Source: CAD feature listing. Evaluate the final solid. Frame: model axes, mm. A direction names the side the tool comes from. Round coordinates to 2 decimals unless told otherwise and drop trailing zeros. Write each loop counter-clockwise with the first axis right and the second up, starting at its lowest first coordinate (ties: lowest second). Pieces come first, ordered by that corner, then holes. Notation, with made-up numbers: M 25.25,-3.5 L 81.25,-3.5 A9 cw 81.25,2.5 Z; hole C 52,39 d8. An arc over 180 degrees is marked long. Answer in a Markdown table with one row per item.
from build123d import *

# Parameters (mm, degrees)
BOSS_EXTRUDE1_DEPTH = 20


with BuildPart() as part:
    # Sketch1 → Boss-Extrude1 (new body)
    with BuildSketch(Plane(origin=(0, 10, 0), x_dir=(1, 0, 0), z_dir=(0, 1, 0))):
        with BuildLine():
            Line((324.62395369, 187.030739377), (-95.643756342, 187.030739377))
            Line((-95.643756342, 187.030739377), (-95.643756342, -106.347051638))
            Line((-95.643756342, -106.347051638), (-65.143756342, -106.347051638))
            Line((-65.143756342, -106.347051638), (-65.143756342, -33.38491726))
            Line((-65.143756342, -33.38491726), (-65.143756342, 39.577217118))
            Line((-65.143756342, 39.577217118), (-65.143756342, 113.493168526))
            ThreePointArc((-65.143756342, 113.493168526), (-65.012374488, 114.20609645), (-64.635490117, 114.825358582))
            Line((-64.635490117, 114.825358582), (-32.303983997, 151.028901364))
            ThreePointArc((-32.303983997, 151.028901364), (-25.878259507, 159.012700556), (-18.37604631, 152.030739377))
            ThreePointArc((-18.37604631, 152.030739377), (-20.50295437, 147.005505557), (-25.591182009, 145.034046113))
            Line((-25.591182009, 145.034046113), (-55.635490117, 111.391617273))
            ThreePointArc((-55.635490117, 111.391617273), (-56.012374488, 110.772355142), (-56.143756342, 110.059427218))
            Line((-56.143756342, 110.059427218), (-56.143756342, 54.882804578))
            ThreePointArc((-56.143756342, 54.882804578), (-54.925540994, 53.041931753), (-52.754943584, 53.443638458))
            Line((-52.754943584, 53.443638458), (-29.527180359, 75.858711639))
            ThreePointArc((-29.527180359, 75.858711639), (-22.786771169, 83.339716759), (-15.544017337, 76.34392727))
            ThreePointArc((-15.544017337, 76.34392727), (-17.860778034, 71.141305851), (-23.277522947, 69.382464097))
            Line((-23.277522947, 69.382464097), (-55.5325691, 38.255953421))
            ThreePointArc((-55.5325691, 38.255953421), (-55.984629167, 37.598571952), (-56.143756342, 36.816787301))
            Line((-56.143756342, 36.816787301), (-56.143756342, -16.173695516))
            ThreePointArc((-56.143756342, -16.173695516), (-54.850365584, -18.044712186), (-52.643052963, -17.495773188))
            Line((-52.643052963, -17.495773188), (-32.564764827, 5.295289321))
            ThreePointArc((-32.564764827, 5.295289321), (-26.169560776, 13.324151457), (-18.643756342, 6.34392727))
            ThreePointArc((-18.643756342, 6.34392727), (-20.753710482, 1.335189757), (-25.811599623, -0.6540602))
            Line((-25.811599623, -0.6540602), (-55.644459721, -34.517633364))
            ThreePointArc((-55.644459721, -34.517633364), (-56.014773012, -35.133101793), (-56.143756342, -35.839711035))
            Line((-56.143756342, -35.839711035), (-56.143756342, -106.347051638))
            Line((-56.143756342, -106.347051638), (39.856243658, -106.347051638))
            Line((39.856243658, -106.347051638), (39.856243658, -33.38491726))
            Line((39.856243658, -33.38491726), (39.856243658, 39.577217118))
            Line((39.856243658, 39.577217118), (39.856243658, 113.493168526))
            ThreePointArc((39.856243658, 113.493168526), (39.987625512, 114.20609645), (40.364509883, 114.825358582))
            Line((40.364509883, 114.825358582), (72.696016003, 151.028901364))
            ThreePointArc((72.696016003, 151.028901364), (79.121740493, 159.012700556), (86.62395369, 152.030739377))
            ThreePointArc((86.62395369, 152.030739377), (84.49704563, 147.005505557), (79.408817991, 145.034046113))
            Line((79.408817991, 145.034046113), (49.364509883, 111.391617273))
            ThreePointArc((49.364509883, 111.391617273), (48.987625512, 110.772355142), (48.856243658, 110.059427218))
            Line((48.856243658, 110.059427218), (48.856243658, 54.882804578))
            ThreePointArc((48.856243658, 54.882804578), (50.074459006, 53.041931753), (52.245056416, 53.443638458))
            Line((52.245056416, 53.443638458), (75.472819641, 75.858711639))
            ThreePointArc((75.472819641, 75.858711639), (82.213228831, 83.339716759), (89.455982663, 76.34392727))
            ThreePointArc((89.455982663, 76.34392727), (87.139221966, 71.141305851), (81.722477053, 69.382464097))
            Line((81.722477053, 69.382464097), (49.4674309, 38.255953421))
            ThreePointArc((49.4674309, 38.255953421), (49.015370833, 37.598571952), (48.856243658, 36.816787301))
            Line((48.856243658, 36.816787301), (48.856243658, -16.173695516))
            ThreePointArc((48.856243658, -16.173695516), (50.149634416, -18.044712186), (52.356947037, -17.495773188))
            Line((52.356947037, -17.495773188), (72.435235173, 5.295289321))
            ThreePointArc((72.435235173, 5.295289321), (78.830439224, 13.324151457), (86.356243658, 6.34392727))
            ThreePointArc((86.356243658, 6.34392727), (84.246289518, 1.335189757), (79.188400377, -0.6540602))
            Line((79.188400377, -0.6540602), (49.355540279, -34.517633364))
            ThreePointArc((49.355540279, -34.517633364), (48.985226988, -35.133101793), (48.856243658, -35.839711035))
            Line((48.856243658, -35.839711035), (48.856243658, -106.347051638))
            Line((48.856243658, -106.347051638), (144.856243658, -106.347051638))
            Line((144.856243658, -106.347051638), (144.856243658, -33.38491726))
            Line((144.856243658, -33.38491726), (144.856243658, 39.577217118))
            Line((144.856243658, 39.577217118), (144.856243658, 113.493168526))
            ThreePointArc((144.856243658, 113.493168526), (144.987625512, 114.20609645), (145.364509883, 114.825358582))
            Line((145.364509883, 114.825358582), (177.696016003, 151.028901364))
            ThreePointArc((177.696016003, 151.028901364), (184.121740493, 159.012700556), (191.62395369, 152.030739377))
            ThreePointArc((191.62395369, 152.030739377), (189.49704563, 147.005505557), (184.408817991, 145.034046113))
            Line((184.408817991, 145.034046113), (154.364509883, 111.391617273))
            ThreePointArc((154.364509883, 111.391617273), (153.987625512, 110.772355142), (153.856243658, 110.059427218))
            Line((153.856243658, 110.059427218), (153.856243658, 54.882804578))
            ThreePointArc((153.856243658, 54.882804578), (155.074459006, 53.041931753), (157.245056416, 53.443638458))
            Line((157.245056416, 53.443638458), (180.472819641, 75.858711639))
            ThreePointArc((180.472819641, 75.858711639), (187.213228831, 83.339716759), (194.455982663, 76.34392727))
            ThreePointArc((194.455982663, 76.34392727), (192.139221966, 71.141305851), (186.722477053, 69.382464097))
            Line((186.722477053, 69.382464097), (154.4674309, 38.255953421))
            ThreePointArc((154.4674309, 38.255953421), (154.015370833, 37.598571952), (153.856243658, 36.816787301))
            Line((153.856243658, 36.816787301), (153.856243658, -16.173695516))
            ThreePointArc((153.856243658, -16.173695516), (155.149634416, -18.044712186), (157.356947037, -17.495773188))
            Line((157.356947037, -17.495773188), (177.435235173, 5.295289321))
            ThreePointArc((177.435235173, 5.295289321), (183.830439224, 13.324151457), (191.356243658, 6.34392727))
            ThreePointArc((191.356243658, 6.34392727), (189.246289518, 1.335189757), (184.188400377, -0.6540602))
            Line((184.188400377, -0.6540602), (154.355540279, -34.517633364))
            ThreePointArc((154.355540279, -34.517633364), (153.985226988, -35.133101793), (153.856243658, -35.839711035))
            Line((153.856243658, -35.839711035), (153.856243658, -106.347051638))
            Line((153.856243658, -106.347051638), (249.856243658, -106.347051638))
            Line((249.856243658, -106.347051638), (249.856243658, -33.38491726))
            Line((249.856243658, -33.38491726), (249.856243658, 39.577217118))
            Line((249.856243658, 39.577217118), (249.856243658, 113.493168526))
            ThreePointArc((249.856243658, 113.493168526), (249.987625512, 114.20609645), (250.364509883, 114.825358582))
            Line((250.364509883, 114.825358582), (282.696016003, 151.028901364))
            ThreePointArc((282.696016003, 151.028901364), (289.121740493, 159.012700556), (296.62395369, 152.030739377))
            ThreePointArc((296.62395369, 152.030739377), (294.49704563, 147.005505557), (289.408817991, 145.034046113))
            Line((289.408817991, 145.034046113), (259.364509883, 111.391617273))
            ThreePointArc((259.364509883, 111.391617273), (258.987625512, 110.772355142), (258.856243658, 110.059427218))
            Line((258.856243658, 110.059427218), (258.856243658, 54.882804578))
            ThreePointArc((258.856243658, 54.882804578), (260.074459006, 53.041931753), (262.245056416, 53.443638458))
            Line((262.245056416, 53.443638458), (285.472819641, 75.858711639))
            ThreePointArc((285.472819641, 75.858711639), (292.213228831, 83.339716759), (299.455982663, 76.34392727))
            ThreePointArc((299.455982663, 76.34392727), (297.139221966, 71.141305851), (291.722477053, 69.382464097))
            Line((291.722477053, 69.382464097), (259.4674309, 38.255953421))
            ThreePointArc((259.4674309, 38.255953421), (259.015370833, 37.598571952), (258.856243658, 36.816787301))
            Line((258.856243658, 36.816787301), (258.856243658, -16.173695516))
            ThreePointArc((258.856243658, -16.173695516), (260.149634416, -18.044712186), (262.356947037, -17.495773188))
            Line((262.356947037, -17.495773188), (282.435235173, 5.295289321))
            ThreePointArc((282.435235173, 5.295289321), (288.830439224, 13.324151457), (296.356243658, 6.34392727))
            ThreePointArc((296.356243658, 6.34392727), (294.246289518, 1.335189757), (289.188400377, -0.6540602))
            Line((289.188400377, -0.6540602), (259.355540279, -34.517633364))
            ThreePointArc((259.355540279, -34.517633364), (258.985226988, -35.133101793), (258.856243658, -35.839711035))
            Line((258.856243658, -35.839711035), (258.856243658, -106.347051638))
            Line((258.856243658, -106.347051638), (324.62395369, -106.347051638))
            Line((324.62395369, -106.347051638), (324.62395369, 187.030739377))
        make_face()
    extrude(amount=BOSS_EXTRUDE1_DEPTH)


solid = part.part
Q1. Pull-direction query (Z, two-part tool) for faces 1 (the flat face through (169.48, 19.86, 17.35)), 2 (the flat face through (324.624, 20, -38)), 3 (the flat face through (-9, 20, 106.347)); classes: pulls with the +Z half, pulls with the -Z half, needs draft (parallel to the pull), parting line crosses it, or undercut.
Solutions:
| item | result |
|---|---|
| face 1 | undercut |
| face 2 | needs draft |
| face 3 | pulls with the +Z half |
Q2. Access query for faces 4 (the flat face through (56.3, 19.86, -132.67)), 5 (the flat face through (258.856, 20, -83)). Directions: +Z, -Z, +X, -X, +Y, -Y. A direction counts if a zero-diameter tool reaches every point of the face in a straight line with its end or side. Return the directions, or none.
Solutions:
| item | result |
|---|---|
| face 4 | +Y, -Y |
| face 5 | +Z, +Y, -Y |
Q3. Material intervals for probe 1 along X at (y, z) = (26, -95.5); probe 2 along Z at (x, y) = (60.5, 27.5); probe 3 along Z at (x, y) = (81.5, 16.5), sorted ascending.
Solutions:
| item | result |
|---|---|
| probe 1 | x = -95.64 to -65.14, -56.14 to 39.86, 48.86 to 144.86, 153.86 to 249.86, 258.86 to 324.62 |
| probe 2 | z = -187.03 to -137.37, -123.86 to -61.41, -48.9 to 8.25, 21.87 to 106.35 |
| probe 3 | z = -187.03 to -158.77, -145.29 to -83.28, -69.17 to -13.01, 0.32 to 106.35 |
Q4. Section A-A (z = -20.5). Return loops of the section in (x, y), and give its area (3 significant figures).
Solutions:
| item | result |
|---|---|
| outline | M -95.64,10 L -65.14,10 L -65.14,30 L -95.64,30 Z; M -56.14,10 L 39.86,10 L 39.86,30 L -56.14,30 Z; M 48.86,10 L 144.86,10 L 144.86,30 L 48.86,30 Z; M 153.86,10 L 249.86,10 L 249.86,30 L 153.86,30 Z; M 258.86,10 L 324.62,10 L 324.62,30 L 258.86,30 Z |
| area | 7,690 mm2 |
